```python
from build123d import *

# Parameters (mm, degrees)
SKETCH1_W           = 170
SKETCH1_H           = 150
BOSS_EXTRUDE1_DEPTH = 10
BOSS_EXTRUDE2_DEPTH = 170
FILLET1_R           = 10
SHELL1_T            = -2
SKETCH3_W           = 115
SKETCH3_H           = 90
CUT_EXTRUDE1_DEPTH  = 2
SKETCH4_W           = 119
SKETCH4_H           = 94
SKETCH4_W_2         = 115
SKETCH4_H_2         = 90
BOSS_EXTRUDE3_DEPTH = 10
SKETCH5_W           = 119
SKETCH5_H           = 94
BOSS_EXTRUDE4_DEPTH = 2
SKETCH6_R           = 2.5
CUT_EXTRUDE2_DEPTH  = 2
SKETCH7_R           = 6
CUT_EXTRUDE3_DEPTH  = 2


with BuildPart() as part:
    # Sketch1 → Boss-Extrude1 (new body)
    with BuildSketch(Plane(origin=(0, 0, 0), x_dir=(1, 0, 0), z_dir=(0, 1, 0))):
        Rectangle(SKETCH1_W, SKETCH1_H)
    extrude(amount=BOSS_EXTRUDE1_DEPTH)

    # Sketch2 → Boss-Extrude2 (add)
    with BuildSketch(Plane.ZY.offset(85)):
        Polygon((-75, 10), (-75, 50.192378865), (75, 10), align=None)
    extrude(amount=-BOSS_EXTRUDE2_DEPTH)

    # Fillet1
    fillet1_edges = [part.edges().sort_by_distance(p)[0] for p in [
        (0, 50.192378865, -75),
        (-85, 30.096189432, 0),
        (85, 30.096189432, 0),
        (0, 10, 75),
        (85, 5, 75),
        (-85, 5, 75),
        (-85, 25.096189432, -75),
        (85, 25.096189432, -75),
    ]]
    fillet(fillet1_edges, radius=FILLET1_R)

    # Shell1
    shell1_openings = [part.faces().sort_by_distance(p)[0] for p in [
        (0, 0, 0),
    ]]
    offset(amount=SHELL1_T, openings=shell1_openings, kind=Kind.INTERSECTION)

    # Sketch3 → Cut-Extrude1 (cut)
    with BuildSketch(Plane(origin=(0, 28.080127019, 7.524047358), x_dir=(1, 0, 0), z_dir=(0, 0.96592582628907, 0.25881904510251436))):
        with Locations((0, 10)):
            Rectangle(SKETCH3_W, SKETCH3_H)
    extrude(amount=-CUT_EXTRUDE1_DEPTH, mode=Mode.SUBTRACT)

    # Sketch4 → Boss-Extrude3 (add)
    with BuildSketch(Plane(origin=(0, 26.148275366, 7.006409268), x_dir=(1, 0, 0), z_dir=(0, -0.96592582628907, -0.25881904510251436))):
        with Locations((0, -10)):
            Rectangle(SKETCH4_W, SKETCH4_H)
        with Locations((0, -10)):
            Rectangle(SKETCH4_W_2, SKETCH4_H_2, mode=Mode.SUBTRACT)
    extrude(amount=BOSS_EXTRUDE3_DEPTH)

    # Sketch5 → Boss-Extrude4 (add)
    with BuildSketch(Plane(origin=(0, 16.489017103, 4.418218817), x_dir=(1, 0, 0), z_dir=(0, -0.96592582628907, -0.25881904510251436))):
        with Locations((0, -10)):
            Rectangle(SKETCH5_W, SKETCH5_H)
    extrude(amount=BOSS_EXTRUDE4_DEPTH)

    # Sketch6 → Cut-Extrude2 (cut)
    with BuildSketch(Plane(origin=(0, 28.080127019, 7.524047358), x_dir=(1, 0, 0), z_dir=(0, 0.96592582628907, 0.25881904510251436))):
        with Locations(Location((-62.5, 10, 0), (0, 0, 270))):
            Circle(SKETCH6_R)
        with Locations(Location((-62.5, 40, 0), (0, 0, 270))):
            Circle(SKETCH6_R)
        with Locations(Location((-62.5, -20, 0), (0, 0, 270))):
            Circle(SKETCH6_R)
        with Locations(Location((62.5, -20, 0), (0, 0, 270))):
            Circle(SKETCH6_R)
        with Locations(Location((62.5, 40, 0), (0, 0, 270))):
            Circle(SKETCH6_R)
        with Locations(Location((62.5, 10, 0), (0, 0, 270))):
            Circle(SKETCH6_R)
    extrude(amount=-CUT_EXTRUDE2_DEPTH, mode=Mode.SUBTRACT)

    # Sketch7 → Cut-Extrude3 (cut)
    with BuildSketch(Plane(origin=(0, 28.080127019, 7.524047358), x_dir=(1, 0, 0), z_dir=(0, 0.96592582628907, 0.25881904510251436))):
        with Locations(Location((-12.5, -48.59148832, 0), (0, 0, 270))):
            Circle(SKETCH7_R)
        with Locations(Location((12.5, -48.59148832, 0), (0, 0, 270))):
            Circle(SKETCH7_R)
        with Locations(Location((37.5, -48.59148832, 0), (0, 0, 270))):
            Circle(SKETCH7_R)
        with Locations(Location((-37.5, -48.59148832, 0), (0, 0, 270))):
            Circle(SKETCH7_R)
    extrude(amount=-CUT_EXTRUDE3_DEPTH, mode=Mode.SUBTRACT)


solid = part.part
```
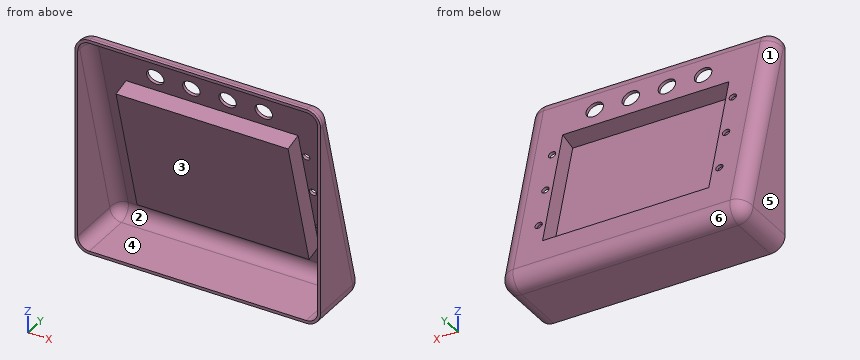
Could you check a few things on this model? Use its own coordinates, in mm. Face numbers are marked on the shaded views. A direction names the side the tool comes from. Coordinates: 2 decimals unless noted, no trailing zeros. Write each loop counter-clockwise with the first axis right and the second up, starting at its lowest first coordinate (ties: lowest second). Pieces come first, ordered by that corner, then holes. Notation, with made-up numbers: (53.5, -34.75) -> (82.5, -34.75) arc R25 cw to (82.5, -3.75) -> close; hole circle Ø8 at (48.5, 3). An arc over 180 degrees is marked (long way). Write item = value, one per line. Start each with the question number.
(1) We'd pull the mould along Z, two halves only. Please class the marked faces 3, 4, 5 and 6: released by +Z, released by -Z, zero draft, split by the parting line, or undercut.
(2) Which directions (+Z, -Z, +X, -X, +Y, -Y) give clear straight access to the entire face, cutting with the end or side of a thin tool? Please do the marked faces 1 and 2.
(3) I need wall thicknesses on line 1 (X direction, y = 17.5, z = -2); line 2 (X direction, y = 24, z = -23); line 3 (X direction, y = 5, z = -64.5). Which ranges of each line are inside material? Lowest first, please. Write a range as [from, to].
(4) I want a section at B-B (x = 28). Please give me the cut outline in (y, z).
(5) Will these pins go through, and if not, where does the flat tip stop? pin 1 (12 mm diameter, centred on x = -43.5, z = -56.5, fed in from -Y); pin 2 (5 mm diameter, centred on y = 28, z = -6.5, fed in from -X); pin 3 (5 mm diameter, centred on x = 57, y = 10.5, fed in from +Z); pin 4 (18.5 mm diameter, centred on x = 34, y = 11, fed in from +Z).
(6) I want a section at A-A (x = 9). Please give me the cut outline in (y, z), plus the area to 3 significant figures.
Result set:
q1.face_3 = undercut
q1.face_4 = undercut
q1.face_5 = zero draft
q1.face_6 = split by the parting line
q2.face_1 = +Z, -X, +Y
q2.face_2 = -Y
q3.line_1 = [-85, -83], [-59.5, 59.5], [83, 85]
q3.line_2 = [-85, -83], [-59.5, -57.5], [57.5, 59.5], [83, 85]
q3.line_3 = [-85, -83], [83, 85]
q4.outline = (0, -75) -> (37.16, -75) arc R10 ccw to (46.82, -62.41) -> (42.32, -45.6) -> (30.72, -48.71) -> (7.43, 38.23) -> (19.02, 41.33) -> (11.99, 67.59) arc R10 ccw to (2.33, 75) -> (0, 75) -> (0, 73) -> (2.33, 73) arc R8 cw to (10.05, 67.07) -> (16.57, 42.75) -> (4.98, 39.64) -> (29.31, -51.16) -> (40.9, -48.05) -> (44.89, -62.93) arc R8 cw to (37.16, -73) -> (0, -73) -> close
q5.pin_1 = 29.13
q5.pin_2 = -84.25
q5.pin_3 = 73.23
q5.pin_4 = 75
q6.outline = (0, -75) -> (37.16, -75) arc R10 ccw to (46.82, -62.41) -> (42.32, -45.6) -> (30.72, -48.71) -> (7.43, 38.23) -> (19.02, 41.33) -> (16.77, 49.75) -> (14.83, 49.23) -> (16.57, 42.75) -> (4.98, 39.64) -> (29.31, -51.16) -> (40.9, -48.05) -> (44.89, -62.93) arc R8 cw to (37.16, -73) -> (0, -73) -> close; (0, 73) -> (2.33, 73) arc R8 cw to (10.05, 67.07) -> (12.31, 58.65) -> (14.24, 59.17) -> (11.99, 67.59) arc R10 ccw to (2.33, 75) -> (0, 75) -> close
q6.area = 433 mm2
